from build123d import *

# Parameters (mm, degrees)
SKETCH1_W           = 175
SKETCH1_H           = 85
BOSS_EXTRUDE1_DEPTH = 2.5
SKETCH2_W           = 85
SKETCH2_H           = 40
CUT_EXTRUDE1_DEPTH  = 2.5
SKETCH3_W           = 175
SKETCH3_H           = 2.5
BOSS_EXTRUDE2_DEPTH = 18.5
SKETCH4_W           = 175
SKETCH4_H           = 15.004979699
BOSS_EXTRUDE3_DEPTH = 2.5


with BuildPart() as part:
    # Sketch1 → Boss-Extrude1 (new body)
    with BuildSketch(Plane(origin=(0, 0, 0), x_dir=(1, 0, 0), z_dir=(0, 1, 0))):
        Rectangle(SKETCH1_W, SKETCH1_H)
    extrude(amount=BOSS_EXTRUDE1_DEPTH)

    # Sketch2 → Cut-Extrude1 (cut)
    with BuildSketch(Plane.XZ):
        with Locations((-42.5, -20)):
            Rectangle(SKETCH2_W, SKETCH2_H)
    extrude(amount=-CUT_EXTRUDE1_DEPTH, mode=Mode.SUBTRACT)

    # Sketch3 → Boss-Extrude2 (add)
    with BuildSketch(Plane(origin=(0, 2.5, 0), x_dir=(1, 0, 0), z_dir=(0, 1, 0))):
        with Locations((0, -41.25)):
            Rectangle(SKETCH3_W, SKETCH3_H)
    extrude(amount=BOSS_EXTRUDE2_DEPTH)

    # Sketch4 → Boss-Extrude3 (add)
    with BuildSketch(Plane(origin=(0, 21, 0), x_dir=(1, 0, 0), z_dir=(0, 1, 0))):
        with Locations((0, -34.99751015)):
            Rectangle(SKETCH4_W, SKETCH4_H)
    extrude(amount=BOSS_EXTRUDE3_DEPTH)


solid = part.part
Part model, mm, in its own coordinate system. A direction names the side the tool comes from. Give positions to 0.01 mm unless a question says otherwise; leave off trailing zeros. Write each loop counter-clockwise with the first axis right and the second up, starting at its lowest first coordinate (ties: lowest second). Pieces come first, ordered by that corner, then holes.
1) Cut at A-A on x = -56.5. Write the cut outline in (y, z).
Resolved:
outline: (0, -42.5) - (2.5, -42.5) - (2.5, -40) - (0, -40) - close; (0, 0) - (2.5, 0) - (2.5, 40) - (21, 40) - (21, 27.5) - (23.5, 27.5) - (23.5, 42.5) - (0, 42.5) - close
2) Cut at B-B on z = -13. Write the cut outline in (x, y), then the cut area to 3 significant figures.
Resolved:
outline: (-87.5, 0) - (-85, 0) - (-85, 2.5) - (-87.5, 2.5) - close; (0, 0) - (87.5, 0) - (87.5, 2.5) - (0, 2.5) - close
area: 225 mm2
3) Pin check, flat tips, straight feed: pin 1 (4 mm diameter, centred on x = 18.5, y = 7.5, fed in from -Z); pin 2 (8 mm diameter, centred on x = -39, z = 8, fed in from -Y); pin 3 (3 mm diameter, centred on x = 4.5, z = -28, fed in from +Y); pin 4 (2 mm diameter, centred on x = -16.5, y = 22, fed in from -Z) (3 decimals). Stop position of each tip, or through.
Resolved:
pin 1: stops at z = 40
pin 2: stops at y = 0
pin 3: stops at y = 2.5
pin 4: stops at z = 27.495
4) Cut at C-C on x = 29. Write the cut outline in (y, z), then the cut area to 3 significant figures.
Resolved:
outline: (0, -42.5) - (2.5, -42.5) - (2.5, 40) - (21, 40) - (21, 27.5) - (23.5, 27.5) - (23.5, 42.5) - (0, 42.5) - close
area: 296 mm2
5) Cut at D-D on z = 33.5. Write the cut outline in (x, y).
Resolved:
outline: (-87.5, 0) - (87.5, 0) - (87.5, 2.5) - (-87.5, 2.5) - close; (-87.5, 21) - (87.5, 21) - (87.5, 23.5) - (-87.5, 23.5) - close
6) Probe L1, parallel to Z at x = -75.5, y = 2; L2, parallel to Y at x = -39, z = 11; L3, parallel to Z at x = -6, y = 4.25. List the from-to ranges inside material, lowest first.
Resolved:
L1: z = -42.5 to -40, 0 to 42.5
L2: y = 0 to 2.5
L3: z = 40 to 42.5
7) Which spindle directions (+Z, -Z, +X, -X, +Y, -Y) get a long thin tool onto all of the face, cutting with end or side? Do faces 1 (the face through (-1, 12, 40)), 2 (the face through (-1, 23.5, 35)). Say none if no direction does.
Resolved:
face 1: -Z, +X, -X
face 2: +Z, -Z, +X, -X, +Y
